from build123d import *

# Parameters (mm, degrees)
SKETCH1_R           = 12.954
BOSS_EXTRUDE2_DEPTH = 38.1
SKETCH2_R           = 0.79375
CUT_EXTRUDE1_DEPTH  = 38.1
CUT_EXTRUDE3_DEPTH  = 1.905


with BuildPart() as part:
    # Sketch1 → Boss-Extrude2 (new body)
    with BuildSketch(Plane(origin=(0, 0, 0), x_dir=(0, 1, 0), z_dir=(0, 0, 1))):
        Polygon((12.85291169, -14.079871961), (18.619982645, 4.091012056), (5.767070955, 18.170884016), (-12.85291169, 14.079871961), (-18.619982645, -4.091012056), (-5.767070955, -18.170884016), align=None)
        with Locations(Location((0, 0, 0), (0, 0, 90))):
            Circle(SKETCH1_R, mode=Mode.SUBTRACT)
    extrude(amount=BOSS_EXTRUDE2_DEPTH)

    # Sketch2 → Cut-Extrude1 (cut)
    with BuildSketch(Plane.XY.offset(38.1)):
        with Locations((-13.57512855, 5.387198703)):
            Circle(SKETCH2_R)
        with Locations((-12.036007248, 8.272880667)):
            Circle(SKETCH2_R)
        with Locations((-9.893350284, 10.743725851)):
            Circle(SKETCH2_R)
        with Locations((-7.254599427, 12.675835758)):
            Circle(SKETCH2_R)
        with Locations((-4.252072661, 13.97232633)):
            Circle(SKETCH2_R)
        with Locations((-1.036329218, 14.568186117)):
            Circle(SKETCH2_R)
        with Locations((2.2313801, 14.433536221)):
            Circle(SKETCH2_R)
        with Locations((5.387198703, 13.57512855)):
            Circle(SKETCH2_R)
        with Locations((8.272880667, 12.036007248)):
            Circle(SKETCH2_R)
        with Locations((10.743725851, 9.893350284)):
            Circle(SKETCH2_R)
        with Locations((12.675835758, 7.254599427)):
            Circle(SKETCH2_R)
        with Locations((13.97232633, 4.252072661)):
            Circle(SKETCH2_R)
        with Locations((14.568186117, 1.036329218)):
            Circle(SKETCH2_R)
        with Locations((14.433536221, -2.2313801)):
            Circle(SKETCH2_R)
        with Locations((13.57512855, -5.387198703)):
            Circle(SKETCH2_R)
        with Locations((12.036007248, -8.272880667)):
            Circle(SKETCH2_R)
        with Locations((9.893350284, -10.743725851)):
            Circle(SKETCH2_R)
        with Locations((7.254599427, -12.675835758)):
            Circle(SKETCH2_R)
        with Locations((4.252072661, -13.97232633)):
            Circle(SKETCH2_R)
        with Locations((1.036329218, -14.568186117)):
            Circle(SKETCH2_R)
        with Locations((-2.2313801, -14.433536221)):
            Circle(SKETCH2_R)
        with Locations((-5.387198703, -13.57512855)):
            Circle(SKETCH2_R)
        with Locations((-8.272880667, -12.036007248)):
            Circle(SKETCH2_R)
        with Locations((-10.743725851, -9.893350284)):
            Circle(SKETCH2_R)
        with Locations((-12.675835758, -7.254599427)):
            Circle(SKETCH2_R)
        with Locations((-13.97232633, -4.252072661)):
            Circle(SKETCH2_R)
        with Locations((-14.568186117, -1.036329218)):
            Circle(SKETCH2_R)
        with Locations((-14.433536221, 2.2313801)):
            Circle(SKETCH2_R)
    extrude(amount=-CUT_EXTRUDE1_DEPTH, mode=Mode.SUBTRACT)

    # Sketch3 → Cut-Extrude3 (cut, symmetric)
    with BuildSketch(Plane(origin=(0, 0, 19.05), x_dir=(0, -1, 0), z_dir=(0, 0, 1))):
        with BuildLine():
            Line((-12.85291169, 14.079871961), (-8.733513074, 9.56722872))
            ThreePointArc((-8.733513074, 9.56722872), (12.652219652, 2.779829827), (-3.918706578, -12.347058547))
            Line((-3.918706578, -12.347058547), (-5.767070955, -18.170884016))
            Line((-5.767070955, -18.170884016), (12.85291169, -14.079871961))
            Line((12.85291169, -14.079871961), (18.619982645, 4.091012056))
            Line((18.619982645, 4.091012056), (5.767070955, 18.170884016))
            Line((5.767070955, 18.170884016), (-12.85291169, 14.079871961))
        make_face()
    extrude(amount=CUT_EXTRUDE3_DEPTH, both=True, mode=Mode.SUBTRACT)


solid = part.part
Here's how the part is built. I have some questions about the finished solid (model axes, mm). Round coordinates to 2 decimals unless told otherwise and drop trailing zeros. One line per question, with ' | ' between items. Start each with the question number.
Q1. We'd pull the mould along Y, two halves only. Please class faces 1 (the flat face through (-15.22, 4.83, 19.08)), 2 (the cylindrical face through (13.41, 6.95, 8.69)), 3 (the flat face through (5.122, 15.696, 18.783)): +Y half, -Y half, draft (parallel to the pull), parting line (faces both ways), or undercut.
Q2. Please list where these lines run through material, in increasing order: line 1 (X direction, y = -12, z = 24); line 2 (X direction, y = -9.5, z = 27); line 3 (Y direction, x = -11, z = 25.5). Write a range as [from, to].
Q3. Will these pins go through, and if not, where does the flat tip stop? pin 1 (1.5 mm diameter, centred on y = 2, z = 30, fed in from +X); pin 2 (1.8 mm diameter, centred on x = -2.23, y = -14.43, fed in from +Z); pin 3 (5 mm diameter, centred on y = -11.5, z = 28, fed in from -X); pin 4 (1 mm diameter, centred on x = -8.5, z = 17.5, fed in from +Y).
Q4. I want a section at A-A (z = 27.5). State how many separate pieces and enclosed holes the cut face has, then the cut area to 3 significant figures.
Response values:
1) face 1: -Y half | face 2: undercut | face 3: +Y half
2) line 1: x = [-14.27, -9.07], [-7.48, -4.88], [4.88, 6.84], [7.67, 11.34] | line 2: x = [-14.82, -11.43], [-10.05, -8.81], [8.81, 14.08] | line 3: y = [-13.83, -10.64], [-9.14, -6.84], [6.84, 12.31]
3) pin 1: stops at x = 16.63 | pin 2: stops at z = 38.1 | pin 3: stops at x = -14.93 | pin 4: stops at y = 15.05
4) separate pieces: 1 | enclosed holes: 29 | area: 362 mm²
